from build123d import *

# Parameters (mm, degrees)
SKETCH2_W           = 50
SKETCH2_H           = 24
SKETCH2_W_2         = 46.5
SKETCH2_H_2         = 10.5
SKETCH2_W_3         = 42.5
SKETCH2_H_3         = 11
BOSS_EXTRUDE1_DEPTH = 47.5
CUT_EXTRUDE1_START  = 47.5
SKETCH2_3_W         = 46.5
SKETCH2_3_H         = 10.5
SKETCH2_3_W_2       = 42.5
SKETCH2_3_H_2       = 11
CUT_EXTRUDE1_DEPTH  = 35
SKETCH3_W           = 50
SKETCH3_H           = 10
SKETCH3_R           = 1.75
CUT_EXTRUDE2_DEPTH  = 20
SKETCH3_3_R         = 1.75
CUT_EXTRUDE3_DEPTH  = 24
CUT_EXTRUDE4_REACH  = 72.002
SKETCH4_W           = 12.5
SKETCH4_H           = 10
SKETCH5_W           = 20
SKETCH5_H           = 7.5
CUT_EXTRUDE5_DEPTH  = 2.5
FILLET1_R           = 2.5


with BuildPart() as part:
    # Sketch2 → Boss-Extrude1 (new body)
    # profile 1 of 3: a face of its own
    with BuildSketch(Plane.XY):
        Rectangle(SKETCH2_W, SKETCH2_H)
        with Locations((0, -4.25)):
            Rectangle(SKETCH2_W_2, SKETCH2_H_2, mode=Mode.SUBTRACT)
    # profile 2 of 3: a face of its own
    with BuildSketch(Plane.XY):
        with Locations((0, -4.25)):
            Rectangle(SKETCH2_W_2, SKETCH2_H_2)
    # profile 3 of 3: a face of its own
    with BuildSketch(Plane.XY):
        with Locations((0, 6.5)):
            Rectangle(SKETCH2_W_3, SKETCH2_H_3)
    extrude(amount=BOSS_EXTRUDE1_DEPTH)

    # Sketch2<3> → Cut-Extrude1 (cut)
    with BuildSketch(Plane.XY.offset(CUT_EXTRUDE1_START)):
        with Locations((0, -4.25)):
            Rectangle(SKETCH2_3_W, SKETCH2_3_H)
        with Locations((0, 6.5)):
            Rectangle(SKETCH2_3_W_2, SKETCH2_3_H_2)
    extrude(amount=-CUT_EXTRUDE1_DEPTH, mode=Mode.SUBTRACT)

    # Sketch3 → Cut-Extrude2 (cut)
    # profile 1 of 4: a face of its own
    with BuildSketch(Plane.XZ.offset(12)):
        with Locations((0, 5)):
            Rectangle(SKETCH3_W, SKETCH3_H)
        with Locations((-16.5, 5)):
            Circle(SKETCH3_R, mode=Mode.SUBTRACT)
        with Locations((0, 5)):
            Circle(SKETCH3_R, mode=Mode.SUBTRACT)
        with Locations((16.5, 5)):
            Circle(SKETCH3_R, mode=Mode.SUBTRACT)
    # profile 2 of 4: a face of its own
    with BuildSketch(Plane.XZ.offset(12)):
        with Locations((-16.5, 5)):
            Circle(SKETCH3_R)
    # profile 3 of 4: a face of its own
    with BuildSketch(Plane.XZ.offset(12)):
        with Locations((0, 5)):
            Circle(SKETCH3_R)
    # profile 4 of 4: a face of its own
    with BuildSketch(Plane.XZ.offset(12)):
        with Locations((16.5, 5)):
            Circle(SKETCH3_R)
    extrude(amount=-CUT_EXTRUDE2_DEPTH, mode=Mode.SUBTRACT)

    # Sketch3<3> → Cut-Extrude3 (cut)
    with BuildSketch(Plane.XZ.offset(12)):
        with Locations(Location((-16.5, 5, 0), (0, 0, 270))):
            Circle(SKETCH3_3_R)
        with Locations(Location((0, 5, 0), (0, 0, 270))):
            Circle(SKETCH3_3_R)
        with Locations(Location((16.5, 5, 0), (0, 0, 270))):
            Circle(SKETCH3_3_R)
    extrude(amount=-CUT_EXTRUDE3_DEPTH, mode=Mode.SUBTRACT)

    # Cut-Extrude4: up to this face of the body (flat: up to its plane)
    cut_extrude4_end = Plane(part.part.faces().sort_by_distance((-25, 0.425531915, 27.739361702))[0])
    # Sketch4 → Cut-Extrude4 (cut, up to the picked face)
    with BuildSketch(Plane(origin=(25, 0, 0), x_dir=(0, 0, -1), z_dir=(1, 0, 0)), mode=Mode.PRIVATE) as cut_extrude4_sk1:
        with Locations((-21.25, 7)):
            Rectangle(SKETCH4_W, SKETCH4_H)
    cut_extrude4_tool1 = split(extrude(cut_extrude4_sk1.sketch, amount=-CUT_EXTRUDE4_REACH, mode=Mode.PRIVATE), bisect_by=cut_extrude4_end, keep=Keep.BOTH, mode=Mode.PRIVATE)
    add(cut_extrude4_tool1.solids().sort_by(Axis((25, 7, 21.25), (-1, 0, 0)))[0], mode=Mode.SUBTRACT)

    # Sketch5 → Cut-Extrude5 (cut)
    with BuildSketch(Plane.XY.offset(12.5)):
        with Locations((0, 4.25)):
            Rectangle(SKETCH5_W, SKETCH5_H)
    extrude(amount=-CUT_EXTRUDE5_DEPTH, mode=Mode.SUBTRACT)

    # Fillet1
    fillet1_edges = [part.edges().sort_by_distance(p)[0] for p in [
        (-23.125, 2, 15),
        (-23.125, 2, 27.5),
        (23.125, 2, 15),
        (23.125, 2, 27.5),
        (17.5, 8, 10),
        (-10, 8, 11.25),
        (10, 8, 11.25),
        (10, 0.5, 11.25),
        (-10, 0.5, 11.25),
        (-17.5, 8, 10),
    ]]
    fillet(fillet1_edges, radius=FILLET1_R)


solid = part.part
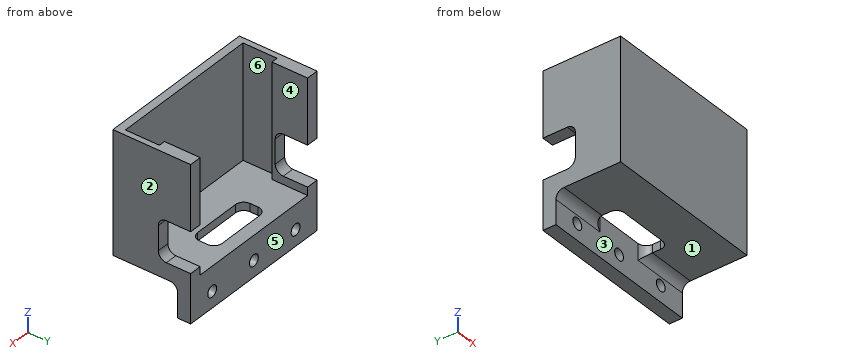
CAD build for the part. Positions are in the model's coordinates, mm. Face numbers are marked on the shaded views. A direction names the side the tool comes from. Give positions to 0.01 mm unless a question says otherwise; leave off trailing zeros. Loops run counter-clockwise (first coordinate to the right, second up) from the corner with the lowest first, then second, coordinate; pieces in that order, holes last. Notation, with made-up numbers: M 86,11 L 92,11 A19 cw 92,42 Z; hole C -1,11.5 d10. An arc over 180 degrees is marked long. Answer in a Markdown table with one row per item. Add a question column.
Item 1: Tool access for the marked faces 4, 5 and 6: list every direction of +Z, -Z, +X, -X, +Y, -Y with a clear straight run to the whole face (end or side of a thin tool).
Item 2: Band-saw the part on C-C on x = 0. Give the cut face in (y, z), then the cut area to 3 significant figures.
Item 3: Drop flat-ended pins along their axis: P1, Ø4, axis at x = -16.5, z = 5, coming from the -Y side; P2, Ø1.9, axis at x = -24, z = 23, coming from the +Y side; P3, Ø1.5, axis at x = -18.5, y = 3.5, coming from the +Z side; P4, Ø10, axis at x = -4.5, y = 7, coming from the -Z side. Give the stop position or say it passes through.
Item 4: Band-saw the part on D-D on y = 6.5. Give the cut face in (x, z).
Item 5: Band-saw the part on A-A on z = 5. Give the cut face in (x, y).
Item 6: Probe probe 1 along X at (y, z) = (9.95, 5); probe 2 along X at (y, z) = (-2, 28); probe 3 along Y at (x, z) = (23, 27). List the from-to ranges inside material, lowest first.
Item 7: Band-saw the part on B-B on x = -5. Give the cut face in (y, z), then the cut area to 3 significant figures.
Item 8: Mould opens along X. For the marked faces 1, 2 and 3 say: +X half, -X half, draft (parallel to the pull), parting line (faces both ways), or undercut.
Reply:
| question | item | result |
|---|---|---|
| 1 | face 4 | +Z, +Y |
| 1 | face 5 | +Z, -Z, +X, -X, +Y |
| 1 | face 6 | +Z |
| 2 | outline | M -12,10 L 0.5,10 L 0.5,12.5 L -9.5,12.5 L -9.5,47.5 L -12,47.5 Z; M 8,0 L 12,0 L 12,3.25 L 8,3.25 Z; M 8,6.75 L 12,6.75 L 12,12.5 L 8,12.5 Z |
| 2 | area | 155 mm^2 |
| 3 | P1 | stops at y = 8 |
| 3 | P2 | stops at y = 2 |
| 3 | P3 | stops at z = 12.5 |
| 3 | P4 | stops at z = 0 |
| 4 | outline | M -25,9.79 L -9.79,9.79 L -9.79,12.5 L -21.25,12.5 L -21.25,15 L -25,15 Z; M -25,27.5 L -21.25,27.5 L -21.25,47.5 L -25,47.5 Z; M 9.79,9.79 L 25,9.79 L 25,15 L 21.25,15 L 21.25,12.5 L 9.79,12.5 Z; M 21.25,27.5 L 25,27.5 L 25,47.5 L 21.25,47.5 Z |
| 5 | outline | M -25,8 L -18.25,8 L -18.25,12 L -25,12 Z; M -14.75,8 L -1.75,8 L -1.75,12 L -14.75,12 Z; M 1.75,8 L 14.75,8 L 14.75,12 L 1.75,12 Z; M 18.25,8 L 25,8 L 25,12 L 18.25,12 Z |
| 6 | probe 1 | x = -25 to -18.25, -14.75 to -1.75, 1.75 to 14.75, 18.25 to 25 |
| 6 | probe 2 | x = -25 to -23.25, 23.25 to 25 |
| 6 | probe 3 | y = -12 to -9.5, 1 to 3 |
| 7 | outline | M -12,10 L 0.5,10 L 0.5,12.5 L -9.5,12.5 L -9.5,47.5 L -12,47.5 Z; M 8,0 L 12,0 L 12,12.5 L 8,12.5 Z |
| 7 | area | 169 mm^2 |
| 8 | face 1 | draft |
| 8 | face 2 | +X half |
| 8 | face 3 | undercut |
